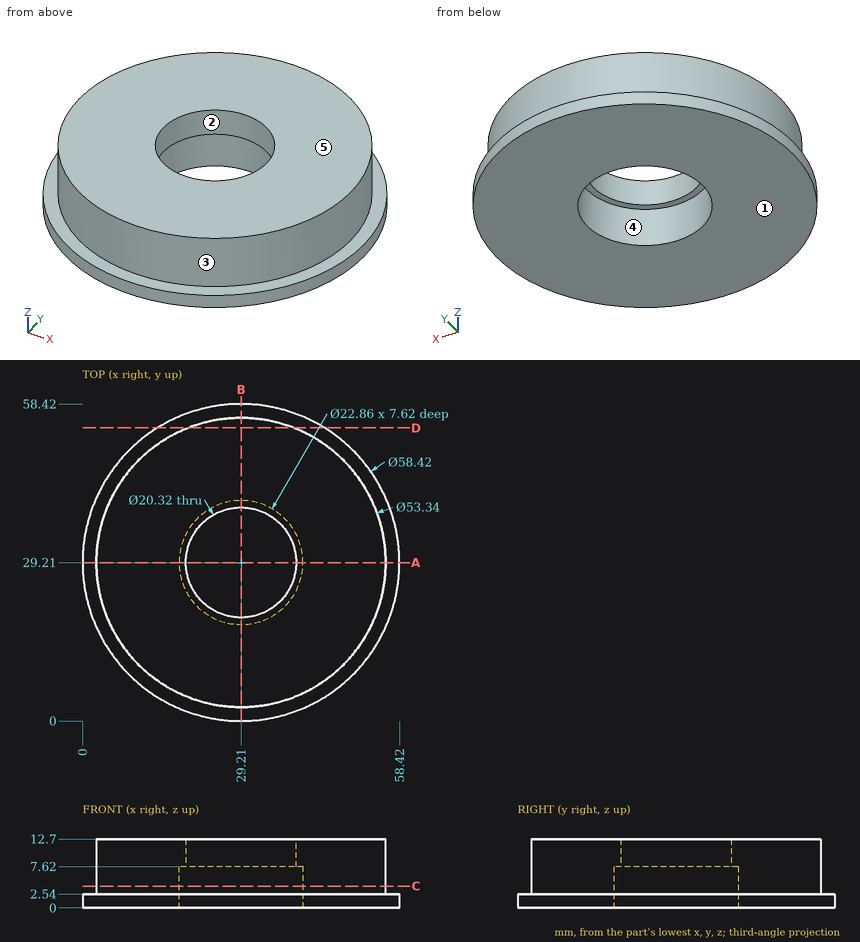
Here's the drawing with two shaded views (mm, measured from the low corner). I have some questions. A direction names the side the tool comes from. Give positions to 0.01 mm unless a question says otherwise; leave off trailing zeros. Loops run counter-clockwise (first coordinate to the right, second up) from the corner with the lowest first, then second, coordinate; pieces in that order, holes last. Notation, with made-up numbers: M 11,5 L 54,5 A9 cw 54,13 Z; hole C -32,49.25 d11. An arc over 180 degrees is marked long. One line per item, written item: value.
1) Imagine slicing it at D-D on y = 54. Write out the boundary of the cut face in (x, z).
Geometry check:
outline: M 13.76,0 L 44.66,0 L 44.66,2.54 L 39.05,2.54 L 39.05,12.7 L 19.37,12.7 L 19.37,2.54 L 13.76,2.54 Z
2) Imagine slicing it at C-C on z = 4. Write out the boundary of the cut face in (x, y), and give its area (3 significant figures).
Geometry check:
outline: C 29.21,29.21 d53.34; hole C 29.21,29.21 d22.86
area: 1,820 mm²
3) On a 3-axis mill with a long thin cutter (end or side, diameter ignored), from which of +Z, -Z, +X, -X, +Y, -Y can I reach the whole of each face in a straight line? I mean the marked faces 4 and 5. Say none if no direction works.
Geometry check:
face 4: -Z
face 5: +Z, +X, -X, +Y, -Y
4) I'm going to push flat-ended pins straight in: pin 1 (5 mm diameter, centred on x = 28, z = 6.5, fed in from +Y); pin 2 (25 mm diameter, centred on x = 28.5, y = 32.5, fed in from -Z); pin 3 (1.5 mm diameter, centred on y = 34, z = 4, fed in from -X); pin 4 (3 mm diameter, centred on x = 29, z = 2.5, fed in from +Y). Where does each tip first touch, or does it pass through?
Geometry check:
pin 1: stops at y = 55.88
pin 2: stops at z = 0
pin 3: stops at x = 2.85
pin 4: stops at y = 58.42
5) Imagine slicing it at A-A on y = 29.21. Write out the boundary of the cut face in (x, z), and give its area (3 significant figures).
Geometry check:
outline: M 0,0 L 17.78,0 L 17.78,7.62 L 19.05,7.62 L 19.05,12.7 L 2.54,12.7 L 2.54,2.54 L 0,2.54 Z; M 39.37,7.62 L 40.64,7.62 L 40.64,0 L 58.42,0 L 58.42,2.54 L 55.88,2.54 L 55.88,12.7 L 39.37,12.7 Z
area: 413 mm²
6) Please list where these lines run through material, in increasing order: line 1 (X direction, y = 29.21, z = 10.2); line 2 (Y direction, x = 29.21, z = 5.5).
Geometry check:
line 1: x = 2.54 to 19.05, 39.37 to 55.88
line 2: y = 2.54 to 17.78, 40.64 to 55.88
7) Thinking about a two-plate mould opening in X: for the marked faces 1, 2 and 3, which applies, +X half, -X half, draft (parallel to the pull), parting line (faces both ways), or undercut?
Geometry check:
face 1: draft
face 2: undercut
face 3: parting line
